Input: part model. Units: mm. Frame: model coordinates. Face numbers are marked on the shaded views. Give positions to 0.01 mm unless a question says otherwise; leave off trailing zeros. Loops run counter-clockwise (first coordinate to the right, second up) from the corner with the lowest first, then second, coordinate; pieces in that order, holes last. Notation, with made-up numbers: (-20, 49) - (19, 49) arc R25 ccw to (19, 88) - close; hole circle Ø9 at (35.25, 19.25). An arc over 180 degrees is marked (long way). Answer as a JSON object with one key per item and string values. Group by question number.
(1) Mould query, pull axis X, two halves, no side actions, for the marked faces 1, 2 and 3. Classes: +X half, -X half, draft (parallel to the pull), parting line (faces both ways), or undercut.
(2) Section query A-A (x = 15.5). Return loops of the section in (y, z).
(3) Section query B-B (y = 336). Return loops of the section in (x, z).
(4) Material intervals for L1, parallel to X at y = 127, z = -55.5; L2, parallel to Y at x = 20, z = -121; L3, parallel to Z at x = 21.25, y = 437, sorted ascending.
(5) Pin query (flat end, axial travel): P1, Ø4, axis at x = 14, z = -168.5, coming from the +Y side; P2, Ø7.5, axis at y = 499.67, z = -220.72, coming from the -X side; P3, Ø5, axis at x = 4, y = 99, coming from the -Z side; P4, Ø6, axis at x = 21.5, y = 390, coming from the -Z side. Return the tip coordinate at first contact, or that it passes through.
(6) Section query C-C (z = -37). Return loops of the section in (x, y), plus the area to 3 significant figures.
Autodesk Inventor part; units mm, degrees
ref_plane "YZ Plane" through (0, 0, 0) normal (1, 0, 0) x (0, 1, 0)
ref_plane "XZ Plane" through (0, 0, 0) normal (0, 1, 0) x (-1, 0, 0)
ref_plane "XY Plane" through (0, 0, 0) normal (0, 0, 1) x (1, 0, 0)
sketch "Sketch1" plane through (0, 0, 0) normal (1, 0, 0) x (0, 1, 0)
  line L0 (0, 0) -> (0, 254)
  line L1 (0, 0) -> (254, 0) construction
  line L2 (0, 0) -> (527.9972, -218.7036)
  line L3 (0, 0) -> (571.5, 0) construction
  line L4 (0, 254) -> (-25.4, 254)
  line L5 (0, 254) -> (25.4, 254) construction
  line L6 (527.9972, -218.7036) -> (518.277, -242.1701)
  line L7 (527.9972, -218.7036) -> (553.3972, -218.7036) construction
  line L8 (518.277, -242.1701) -> (-25.4, -16.9717)
  line L9 (-25.4, -16.9717) -> (-25.4, 254)
  line L10 (-25.4, -16.9717) -> (0, 0)
  dimension "d0" = 254
  dimension "d1" = 90
  dimension "d2" = 571.5
  dimension "d3" = 22.5
  dimension "d4" = 25.4
  dimension "d5" = 180
  dimension "d6" = 25.4
  dimension "d7" = 112.5
  dimension "d8" = 90
extrude "Extrusion3" add sketch "Sketch1" along normal blind 25.4 contours L2 L6 L8 L10
sketch "Sketch3" plane through (0, 527.9972, -218.7036) normal (0, 0.9239, -0.3827) x (1, 0, 0)
  line L0 (0, 25.4) -> (1.5875, 25.4)
  line L1 (1.5875, 25.4) -> (1.5875, 23.8125)
  line L2 (1.5875, 23.8125) -> (0, 23.8125)
  line L3 (0, 23.8125) -> (0, 25.4)
  line L4 (25.4, 0) -> (23.8125, 0)
  line L5 (23.8125, 0) -> (23.8125, 1.5875)
  line L6 (23.8125, 1.5875) -> (25.4, 1.5875)
  line L7 (25.4, 1.5875) -> (25.4, 0)
  line L8 (1.5875, 23.8125) -> (23.8125, 23.8125)
  line L9 (23.8125, 23.8125) -> (23.8125, 1.5875)
  line L10 (23.8125, 1.5875) -> (1.5875, 1.5875)
  line L11 (1.5875, 1.5875) -> (1.5875, 23.8125)
  dimension "d19" = 1.5875
  dimension "d20" = 1.5875
  dimension "d21" = 1.5875
  dimension "d22" = 1.5875
extrude "Extrusion4" cut sketch "Sketch3" against normal blind 2540 contours L8 L9 L10 L11
sketch "Sketch4" plane through (25.4, 0, 0) normal (1, 0, 0) x (0, 0, -1)
  line L0 (242.1701, 518.277) -> (218.7036, 527.9972)
  line L1 (218.7036, 527.9972) -> (0, 0)
  line L2 (230.4369, 523.1371) -> (220.7167, 499.6705)
  line L3 (230.4369, 523.1371) -> (255.8369, 523.1371) construction
  circle A0 centre (220.7167, 499.6705) radius 6.35
  line L4 (220.7167, 499.6705) -> (196.4163, 441.0042)
  circle A1 centre (196.4163, 441.0042) radius 7.112
  dimension "d25" = 25.4
  dimension "d26" = 112.5
  dimension "d27" = 12.7
  dimension "d28" = 63.5
  dimension "d29" = 14.224
extrude "Extrusion5" cut sketch "Sketch4" against normal blind 50.8
properties part number "CatapultArmSquare-Top"
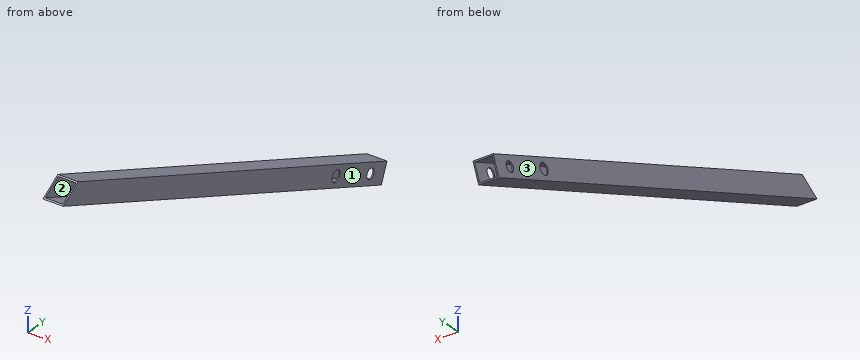
Recorded:
{
 "1": {"face 1": "+X half", "face 2": "undercut", "face 3": "-X half"},
 "2": {"outline": "(-25.4, -16.97) - (518.28, -242.17) - (518.88, -240.7) - (-23.81, -15.91) - close; (-1.59, -1.06) - (527.39, -220.17) - (528, -218.7) - (0, 0) - close"},
 "3": {"outline": "(0, -166.67) - (25.4, -166.67) - (25.4, -139.18) - (0, -139.18) - close; hole (1.59, -164.95) - (23.81, -164.95) - (23.81, -140.89) - (1.59, -140.89) - close"},
 "4": {"L1": "x = 0 to 1.59, 23.81 to 25.4", "L2": "y = 225.75 to 229.89, 287.97 to 292.12", "L3": "z = -208.5 to -206.79, -182.73 to -181.01"},
 "5": {"P1": "stops at y = 411.62", "P2": "passes through", "P3": "stops at z = -69.54", "P4": "stops at z = -190.28"},
 "6": {"outline": "(0, 22.95) - (25.4, 22.95) - (25.4, 89.33) - (0, 89.33) - close; hole (1.59, 27.1) - (23.81, 27.1) - (23.81, 85.18) - (1.59, 85.18) - close", "area": "395 mm^2"}
}
